Autodesk Inventor part; units mm, degrees
ref_plane "to_rail_XY" through (9.5, 17.65, 228.6) normal (0, 0, 1) x (1, 0, 0)
ref_plane "to_rail_YZ" through (9.5, 17.65, 228.6) normal (1, 0, 0) x (0, 1, 0)
ref_plane "to_rail_ZX" through (9.5, 17.65, 228.6) normal (0, 1, 0) x (0, 0, 1)
sketch "Sketch_1" plane through (0, 0, 0) normal (0, 0, 1) x (1, 0, 0)
  line L0 (0, 32.8967) -> (0, 2.4033)
  line L1 (0, 2.4033) -> (6.2112, 0)
  line L2 (6.2112, 0) -> (7.15, 0)
  arc A0 (7.15, 0) -> (9, 1.85) centre (7.15, 1.85) ccw
  line L3 (9, 1.85) -> (9, 2.1444)
  line L4 (9, 2.1444) -> (8.493, 2.1888)
  arc A1 (5.9824, 0.6246) -> (8.493, 2.1888) centre (6.65, 2.35) ccw
  line L5 (5.9824, 0.6246) -> (0.5, 2.7459)
  line L6 (0.5, 2.7459) -> (0.5, 32.5541)
  line L7 (0.5, 32.5541) -> (5.9824, 34.6754)
  arc A2 (8.493, 33.1112) -> (5.9824, 34.6754) centre (6.65, 32.95) ccw
  line L8 (8.493, 33.1112) -> (9, 33.1556)
  line L9 (9, 33.1556) -> (9, 33.45)
  arc A3 (9, 33.45) -> (7.15, 35.3) centre (7.15, 33.45) ccw
  line L10 (7.15, 35.3) -> (6.2112, 35.3)
  line L11 (6.2112, 35.3) -> (0, 32.8967)
extrude "Extrusion1" add sketch "Sketch_1" along normal blind 457.2
sketch "Sketch_4" plane through (0, 0, 0) normal (1, 0, 0) x (0, 1, 0)
  arc A0 (17.65, 332.85) -> (15.4, 330.6) centre (17.65, 330.6) ccw
  line L0 (15.4, 330.6) -> (15.4, 329.8)
  arc A1 (15.4, 329.8) -> (17.65, 327.55) centre (17.65, 329.8) ccw
  arc A2 (17.65, 327.55) -> (19.9, 329.8) centre (17.65, 329.8) ccw
  line L1 (19.9, 329.8) -> (19.9, 330.6)
  arc A3 (19.9, 330.6) -> (17.65, 332.85) centre (17.65, 330.6) ccw
extrude "Extrusion2" cut sketch "Sketch_4" along normal blind 0.5
sketch "Sketch_5" plane through (0, 0, 0) normal (1, 0, 0) x (0, 1, 0)
  arc A0 (17.65, 231.25) -> (15.4, 229) centre (17.65, 229) ccw
  line L0 (15.4, 229) -> (15.4, 228.2)
  arc A1 (15.4, 228.2) -> (17.65, 225.95) centre (17.65, 228.2) ccw
  arc A2 (17.65, 225.95) -> (19.9, 228.2) centre (17.65, 228.2) ccw
  line L1 (19.9, 228.2) -> (19.9, 229)
  arc A3 (19.9, 229) -> (17.65, 231.25) centre (17.65, 229) ccw
extrude "Extrusion3" cut sketch "Sketch_5" along normal blind 0.5
sketch "Sketch_6" plane through (0, 0, 0) normal (1, 0, 0) x (0, 1, 0)
  arc A0 (17.65, 142.35) -> (15.4, 140.1) centre (17.65, 140.1) ccw
  line L0 (15.4, 140.1) -> (15.4, 139.3)
  arc A1 (15.4, 139.3) -> (17.65, 137.05) centre (17.65, 139.3) ccw
  arc A2 (17.65, 137.05) -> (19.9, 139.3) centre (17.65, 139.3) ccw
  line L1 (19.9, 139.3) -> (19.9, 140.1)
  arc A3 (19.9, 140.1) -> (17.65, 142.35) centre (17.65, 140.1) ccw
extrude "Extrusion4" cut sketch "Sketch_6" along normal blind 0.5
sketch "Sketch_7" plane through (0, 0, 0) normal (1, 0, 0) x (0, 1, 0)
  line L0 (18.05, 443.55) -> (17.25, 443.55)
  arc A0 (17.25, 443.55) -> (15, 441.3) centre (17.25, 441.3) ccw
  arc A1 (15, 441.3) -> (17.25, 439.05) centre (17.25, 441.3) ccw
  line L1 (17.25, 439.05) -> (18.05, 439.05)
  arc A2 (18.05, 439.05) -> (20.3, 441.3) centre (18.05, 441.3) ccw
  arc A3 (20.3, 441.3) -> (18.05, 443.55) centre (18.05, 441.3) ccw
extrude "Extrusion5" cut sketch "Sketch_7" along normal blind 0.5
sketch "Sketch_3" plane through (0, 0, 0) normal (1, 0, 0) x (0, 1, 0)
  line L0 (18.05, 30.85) -> (17.25, 30.85)
  arc A0 (17.25, 30.85) -> (15, 28.6) centre (17.25, 28.6) ccw
  arc A1 (15, 28.6) -> (17.25, 26.35) centre (17.25, 28.6) ccw
  line L1 (17.25, 26.35) -> (18.05, 26.35)
  arc A2 (18.05, 26.35) -> (20.3, 28.6) centre (18.05, 28.6) ccw
  arc A3 (20.3, 28.6) -> (18.05, 30.85) centre (18.05, 28.6) ccw
extrude "Extrusion6" cut sketch "Sketch_3" along normal blind 0.5
sketch "Sketch_8" plane through (0, 0, 0) normal (1, 0, 0) x (0, 1, 0)
  line L0 (18.05, 18.15) -> (17.25, 18.15)
  arc A0 (17.25, 18.15) -> (15, 15.9) centre (17.25, 15.9) ccw
  arc A1 (15, 15.9) -> (17.25, 13.65) centre (17.25, 15.9) ccw
  line L1 (17.25, 13.65) -> (18.05, 13.65)
  arc A2 (18.05, 13.65) -> (20.3, 15.9) centre (18.05, 15.9) ccw
  arc A3 (20.3, 15.9) -> (18.05, 18.15) centre (18.05, 15.9) ccw
extrude "Extrusion7" cut sketch "Sketch_8" along normal blind 0.5
sketch "Sketch_9" plane through (0, 0, 0) normal (1, 0, 0) x (0, 1, 0)
  line L0 (18.05, 430.85) -> (17.25, 430.85)
  arc A0 (17.25, 430.85) -> (15, 428.6) centre (17.25, 428.6) ccw
  arc A1 (15, 428.6) -> (17.25, 426.35) centre (17.25, 428.6) ccw
  line L1 (17.25, 426.35) -> (18.05, 426.35)
  arc A2 (18.05, 426.35) -> (20.3, 428.6) centre (18.05, 428.6) ccw
  arc A3 (20.3, 428.6) -> (18.05, 430.85) centre (18.05, 428.6) ccw
extrude "Extrusion8" cut sketch "Sketch_9" along normal blind 0.5
sketch "Sketch_10" plane through (0, 0, 0) normal (1, 0, 0) x (0, 1, 0)
  arc A0 (17.75, 418.55) -> (15.5, 416.3) centre (17.75, 416.3) ccw
  line L0 (15.5, 416.3) -> (15.5, 415.5)
  arc A1 (15.5, 415.5) -> (17.75, 413.25) centre (17.75, 415.5) ccw
  arc A2 (17.75, 413.25) -> (20, 415.5) centre (17.75, 415.5) ccw
  line L1 (20, 415.5) -> (20, 416.3)
  arc A3 (20, 416.3) -> (17.75, 418.55) centre (17.75, 416.3) ccw
extrude "Extrusion9" cut sketch "Sketch_10" along normal blind 0.5
sketch "Sketch10" plane through (0, 2.4033, 0) normal (-1, 0, 0) x (0, 0, 1)
  point P0 (55, 15.2467)
hole "Hole1" at (0, 17.65, 55) direction (1, 0, 0) diameter 9.5 depth 0.5
ref_plane "to_rail_XY" through (9.5, 17.65, 228.6) normal (0, 0, 1) x (1, 0, 0)
ref_plane "to_rail_YZ" through (9.5, 17.65, 228.6) normal (1, 0, 0) x (0, 1, 0)
ref_plane "to_rail_ZX" through (9.5, 17.65, 228.6) normal (0, 1, 0) x (0, 0, 1)
properties part number "body_SSRN3618" material "鉄 灰色"
Source: CAD feature listing. Evaluate the final solid. Frame: model axes, mm. Give positions to 0.01 mm unless a question says otherwise; leave off trailing zeros. Write each loop counter-clockwise with the first axis right and the second up, starting at its lowest first coordinate (ties: lowest second). Pieces come first, ordered by that corner, then holes. Notation, with made-up numbers: M 11,7.25 L 48,7.25 A22 ccw 48,45.25 Z; hole C 1.25,-40 d1. An arc over 180 degrees is marked long. Return JSON: item names as keys, results as strings. Group by question number.
1) Cut plane B-B, the plane x = 3.5. Output: boundary loops of the cut face in (y, z), plus the area to 3 significant figures.
2) Cut plane A-A, the plane z = 55. Output: boundary loops of the cut face in (x, y).
3) Pull-direction query (Y, two-part tool) for faces 1 (the face through (0.254, 22.287, 53.97)), 2 (the face through (0, 18, 225)); classes: pulls with the +Y half, pulls with the -Y half, needs draft (parallel to the pull), parting line crosses it, or undercut.
4) Material intervals for line 1 along Y through (x, z) = (0.1, 55); line 2 along Y through (x, z) = (0.15, 55); line 3 along X through (y, z) = (9.5, 35), sorted ascending. Write a range as [from, to].
5) Cut plane C-C, the plane y = 27.5. Output: boundary loops of the cut face in (x, z), plus the area to 3 significant figures.
6) Pin query (flat end, axial travel): P1, Ø1, axis at y = 13, z = 218.5, coming from the +X side; P2, Ø1, axis at x = 4, z = 103.5, coming from the -Y side; P3, Ø0.6, axis at x = 0.5, z = 330, coming from the -Y side. Return the tip coordinate at first contact, or that it passes through.
Recorded:
{
 "1": {"outline": "M 1.05,0 L 1.59,0 L 1.59,457.2 L 1.05,457.2 Z; M 33.71,0 L 34.25,0 L 34.25,457.2 L 33.71,457.2 Z", "area": "490 mm²"},
 "2": {"outline": "M 0,2.4 L 6.21,0 L 7.15,0 A1.85 ccw 9,1.85 L 9,2.14 L 8.49,2.19 A1.85 cw 5.98,0.62 L 0.5,2.75 L 0.5,12.9 L 0,12.9 Z; M 0,22.4 L 0.5,22.4 L 0.5,32.55 L 5.98,34.68 A1.85 cw 8.49,33.11 L 9,33.16 L 9,33.45 A1.85 ccw 7.15,35.3 L 6.21,35.3 L 0,32.9 Z"},
 "3": {"face 1": "undercut", "face 2": "needs draft"},
 "4": {"line 1": "y = [2.36, 12.9], [22.4, 32.94]", "line 2": "y = [2.35, 12.9], [22.4, 32.95]", "line 3": "x = [0, 0.5]"},
 "5": {"outline": "M 0,0 L 0.5,0 L 0.5,457.2 L 0,457.2 Z", "area": "229 mm²"},
 "6": {"P1": "stops at x = 0.5", "P2": "stops at y = 0.66", "P3": "stops at y = 2.09"}
}
